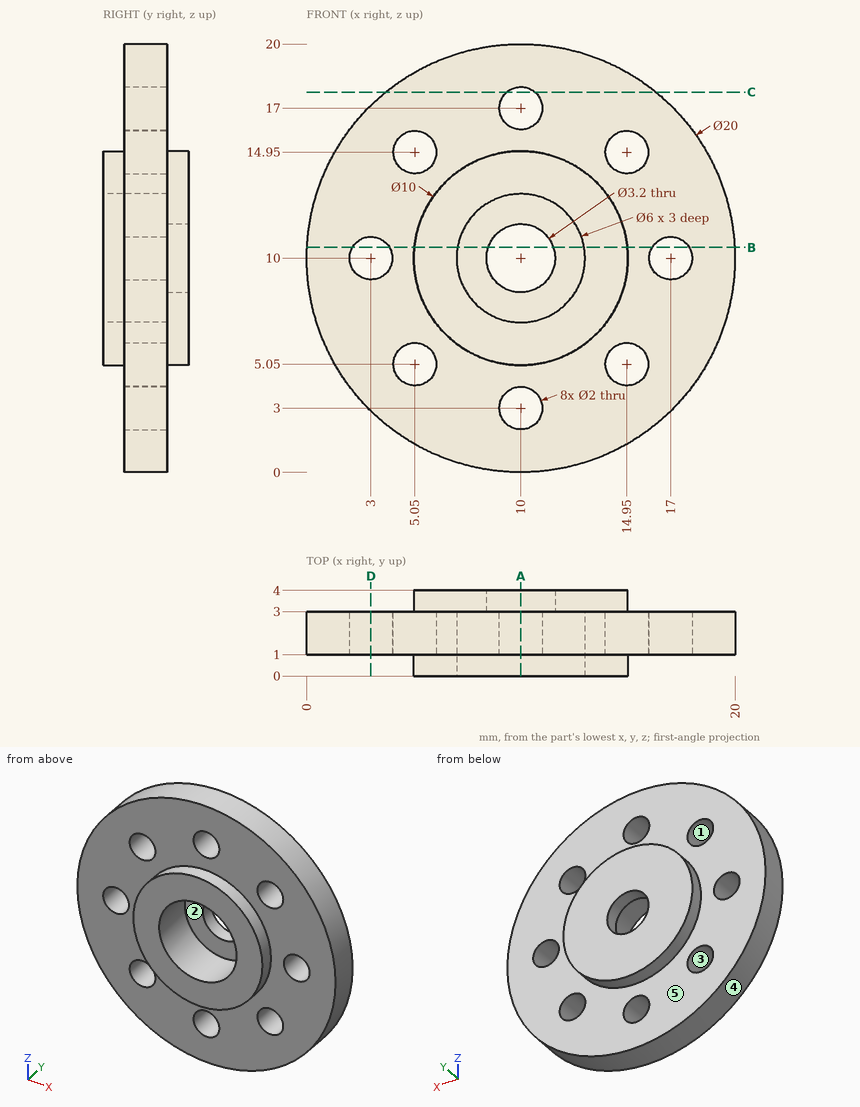
The figure shows three views and two pictorial views of one solid part (mm, origin at its lowest corner). Answer the questions. A direction names the side the tool comes from. Give positions to 0.01 mm unless a question says otherwise; leave off trailing zeros. Loops run counter-clockwise (first coordinate to the right, second up) from the corner with the lowest first, then second, coordinate; pieces in that order, holes last. Notation, with made-up numbers: (78, 34) -> (115, 34) arc R20 cw to (115, 41) -> close; hole circle Ø8 at (-9, -9.5). An arc over 180 degrees is marked (long way). Use a Markdown table: item, result. Add a question column.
1. Section A-A on x = 10 is taken. Determine the outline of the cut face in (y, z), and give its area (3 significant figures).
2. Flat-ended cylindrical pins translate along their axes: pin 1 Ø2.5 at (x, z) = (5.05, 5.05) entering from +Y; pin 2 Ø2.5 at (x, z) = (10, 10) entering from -Y; pin 3 Ø2.5 at (x, z) = (10, 3) entering from -Y; pin 4 Ø5 at (x, z) = (10, 10) entering from -Y. Find the tip coordinate at first contact, or state that the pin passes through.
3. Section D-D on x = 3 is taken. Determine the outline of the cut face in (y, z).
4. Find the intervals of material crossed by probe 1 along Z at (x, y) = (10, 2.5); probe 2 along Z at (x, y) = (10, 3.3); probe 3 along Y at (x, z) = (17.25, 13.5), in increasing order.
5. Determine the mould class of the marked faces 3, 4 and 5 for opening direction X: released by +X, released by -X, zero draft, split by the parting line, or undercut.
6. For the marked faces 1 and 2, determine the directions among +Z, -Z, +X, -X, +Y, -Y from which every point of the face is accessible in a straight line to the end or side of a thin tool.
7. Section B-B on z = 10.5 is taken. Determine the outline of the cut face in (x, y) (1 decimal).
8. Section C-C on z = 17.75 is taken. Determine the outline of the cut face in (x, y).
Results below:
| question | item | result |
|---|---|---|
| 1 | outline | (0, 5) -> (1, 5) -> (1, 4) -> (3, 4) -> (3, 5) -> (4, 5) -> (4, 8.4) -> (3, 8.4) -> (3, 7) -> (0, 7) -> close; (0, 13) -> (3, 13) -> (3, 11.6) -> (4, 11.6) -> (4, 15) -> (3, 15) -> (3, 16) -> (1, 16) -> (1, 15) -> (0, 15) -> close; (1, 0) -> (3, 0) -> (3, 2) -> (1, 2) -> close; (1, 18) -> (3, 18) -> (3, 20) -> (1, 20) -> close |
| 1 | area | 30.8 mm^2 |
| 2 | pin 1 | stops at y = 3 |
| 2 | pin 2 | passes through |
| 2 | pin 3 | stops at y = 1 |
| 2 | pin 4 | stops at y = 3 |
| 3 | outline | (1, 2.86) -> (3, 2.86) -> (3, 9) -> (1, 9) -> close; (1, 11) -> (3, 11) -> (3, 17.14) -> (1, 17.14) -> close |
| 4 | probe 1 | z = 0 to 2, 4 to 7, 13 to 16, 18 to 20 |
| 4 | probe 2 | z = 5 to 8.4, 11.6 to 15 |
| 4 | probe 3 | y = 1 to 3 |
| 5 | face 3 | undercut |
| 5 | face 4 | split by the parting line |
| 5 | face 5 | zero draft |
| 6 | face 1 | +Y, -Y |
| 6 | face 2 | -Y |
| 7 | outline | (0, 1) -> (2.1, 1) -> (2.1, 3) -> (0, 3) -> close; (3.9, 1) -> (5, 1) -> (5, 0) -> (7, 0) -> (7, 3) -> (8.5, 3) -> (8.5, 4) -> (5, 4) -> (5, 3) -> (3.9, 3) -> close; (11.5, 3) -> (13, 3) -> (13, 0) -> (15, 0) -> (15, 1) -> (16.1, 1) -> (16.1, 3) -> (15, 3) -> (15, 4) -> (11.5, 4) -> close; (17.9, 1) -> (20, 1) -> (20, 3) -> (17.9, 3) -> close |
| 8 | outline | (3.68, 1) -> (9.34, 1) -> (9.34, 3) -> (3.68, 3) -> close; (10.66, 1) -> (16.32, 1) -> (16.32, 3) -> (10.66, 3) -> close |
